from build123d import *

# Parameters (mm, degrees)
F1_DEPTH = 30
F0_W     = 30
F0_H     = 12
F2_DEPTH = 5
F3_R     = 4
F4_DEPTH = 40.001
F5_R     = 2.5
F6_DEPTH = 5.001
F7_W     = 5.6
F7_H     = 13.8
F8_DEPTH = 30.001
F0_W_2   = 12
F0_H_2   = 20
F0_R     = 2.5
F9_DEPTH = 5
F10_R    = 4


# Not quite as in the source:
# - a feature names something its author has since deleted; it is built from what else it names


with BuildPart() as f1:
    # F0 (on Top) → F1 (new body)
    with BuildSketch(Plane.XY):
        Polygon((15, -15), (20, -15), (20, 15), (-20, 15), (-20, 10.0191985071), (-20, -9.9808014929), (-20, -15), (-15, -15), align=None)
    extrude(amount=F1_DEPTH)

    # F0 (on Top) → F2 (join)
    with BuildSketch(Plane.XY):
        with Locations((0, -21)):
            Rectangle(F0_W, F0_H)
    extrude(amount=F2_DEPTH)

    # F3 (on face) → F4 (cut, through all)
    with BuildSketch(Plane.YZ.offset(20)):
        with Locations((0, 15)):
            Circle(F3_R)
    extrude(amount=-F4_DEPTH, mode=Mode.SUBTRACT)

    # F5 (on face) → F6 (cut, through all)
    with BuildSketch(Plane.XY.offset(5)):
        with Locations((9, -22.75)):
            Circle(F5_R)
        with Locations((-9, -22.75)):
            Circle(F5_R)
    extrude(amount=-F6_DEPTH, mode=Mode.SUBTRACT)

    # F7 (on face) → F8 (cut, through all)
    with BuildSketch(Plane.XY.offset(30)):
        Rectangle(F7_W, F7_H)
    extrude(amount=-F8_DEPTH, mode=Mode.SUBTRACT)

    # F0 (on Top) → F9 (join)
    with BuildSketch(Plane.XY):
        with Locations((-26, 0.0191985071)):
            Rectangle(F0_W_2, F0_H_2)
        with Locations((-26.2869596481, -5.2162762731)):
            Circle(F0_R, mode=Mode.SUBTRACT)
        with Locations((-26.2869596481, 5.0912299193)):
            Circle(F0_R, mode=Mode.SUBTRACT)
    extrude(amount=F9_DEPTH)

    # F10
    f10_edges = [f1.edges().sort_by_distance(p)[0] for p in [
        (-20, 0.019199, 5),
        (-20, 15, 15),
        (-20, 0, 30),
        (-20, -15, 15),
        (0, -15, 5),
        (0, -15, 30),
        (20, -15, 15),
        (20, 0, 30),
        (0, 15, 30),
        (20, 15, 15),
    ]]
    fillet(f10_edges, radius=F10_R)


solid = f1.part
Could you check a few things on this model? Use its own coordinates, in mm. A direction names the side the tool comes from. Give positions to 0.01 mm unless a question says otherwise; leave off trailing zeros. Order: outer loops, then holes, each group sorted by start corner. A loop starts at its lowest first (then second) coordinate and runs counter-clockwise, first axis right, second up. Notation, with made-up numbers: (59.25, 39) -> (93.25, 39) arc R21 ccw to (93.25, 69) -> close; hole circle Ø10 at (19, -5). An arc over 180 degrees is marked (long way). Return JSON: item names as keys, results as strings.
1. Imagine slicing it at C-C on z = 15. List the corners of the cut face in (x, y) for me, then the cut area to 3 significant figures.
Answer list:
{"outline": "(-20, -11) arc R4 ccw to (-16, -15) -> (16, -15) arc R4 ccw to (20, -11) -> (20, -4) -> (2.8, -4) -> (2.8, -6.9) -> (-2.8, -6.9) -> (-2.8, -4) -> (-20, -4) -> close; (-20, 4) -> (-2.8, 4) -> (-2.8, 6.9) -> (2.8, 6.9) -> (2.8, 4) -> (20, 4) -> (20, 11) arc R4 ccw to (16, 15) -> (-16, 15) arc R4 ccw to (-20, 11) -> close", "area": "834 mm2"}
2. On a 3-axis mill with a long thin cutter (end or side, diameter ignored), from which of +Z, -Z, +X, -X, +Y, -Y can I reach the whole of each face in a straight line? I mean faces 1 (the flat face through (-4, 0, 30)), 2 (the flat face through (-29, 0, 5)), 3 (the flat face through (-15, -21, 2)). Say none if no direction works.
Answer list:
{"face 1": "+Z, +X, -X, +Y, -Y", "face 2": "+Z, -X, +Y, -Y", "face 3": "+Z, -Z, -X, -Y"}
3. For pin 1 Ø6 at (x, y) = (9, -22.75) entering from +Z; pin 2 Ø1.5 at (y, z) = (-22.5, 4) entering from -X; pin 3 Ø13 at (y, z) = (0, 15) entering from -X, each with a flat end and sliding along its axis, tell me the tip position at first contact or that it passes through.
Answer list:
{"pin 1": "stops at z = 5", "pin 2": "stops at x = -15", "pin 3": "stops at x = -20.03"}
4. Thinking about a two-plate mould opening in X: for faces 4 (the flat face through (-2.8, -3, 12)), 5 (the cylindrical face through (0.224, -13.859, 28.797)), 6 (the flat face through (-20, 3, 19)), which applies, pulls with the +X half, pulls with the -X half, needs draft (parallel to the pull), parting line crosses it, or undercut?
Answer list:
{"face 4": "undercut", "face 5": "needs draft", "face 6": "pulls with the -X half"}
5. Imagine slicing it at A-A on x = 10.5. List the corners of the cut face in (y, z) for me, then the cut area to 3 significant figures.
Answer list:
{"outline": "(-27, 0) -> (-24.75, 0) -> (-24.75, 5) -> (-27, 5) -> close; (-20.75, 0) -> (15, 0) -> (15, 26) arc R4 ccw to (11, 30) -> (-11, 30) arc R4 ccw to (-15, 26) -> (-15, 9) arc R4 cw to (-19, 5) -> (-20.75, 5) -> close; hole circle Ø8 at (0, 15)", "area": "886 mm2"}
6. Imagine slicing it at B-B on y = -22.75. List the corners of the cut face in (x, z) for me, then the cut area to 3 significant figures.
Answer list:
{"outline": "(-15, 0) -> (-11.5, 0) -> (-11.5, 5) -> (-15, 5) -> close; (-6.5, 0) -> (6.5, 0) -> (6.5, 5) -> (-6.5, 5) -> close; (11.5, 0) -> (15, 0) -> (15, 5) -> (11.5, 5) -> close", "area": "100 mm2"}
7. I need wall thicknesses on line 1 (X direction, y = 5, z = 23); line 2 (X direction, y = 4, z = 3.5); line 3 (Y direction, x = 9, z = 2). Which ranges of each line are inside material? Lowest first, please. Write a range as from..to.
Answer list:
{"line 1": "x = -20..-2.8, 2.8..20", "line 2": "x = -32..-28.54, -24.04..-2.8, 2.8..20", "line 3": "y = -27..-25.25, -20.25..15"}
8. Imagine slicing it at D-D on x = -1.5. List the corners of the cut face in (y, z) for me, then the cut area to 3 significant figures.
Answer list:
{"outline": "(-27, 0) -> (-6.9, 0) -> (-6.9, 30) -> (-11, 30) arc R4 ccw to (-15, 26) -> (-15, 9) arc R4 cw to (-19, 5) -> (-27, 5) -> close; (6.9, 0) -> (15, 0) -> (15, 26) arc R4 ccw to (11, 30) -> (6.9, 30) -> close", "area": "543 mm2"}
